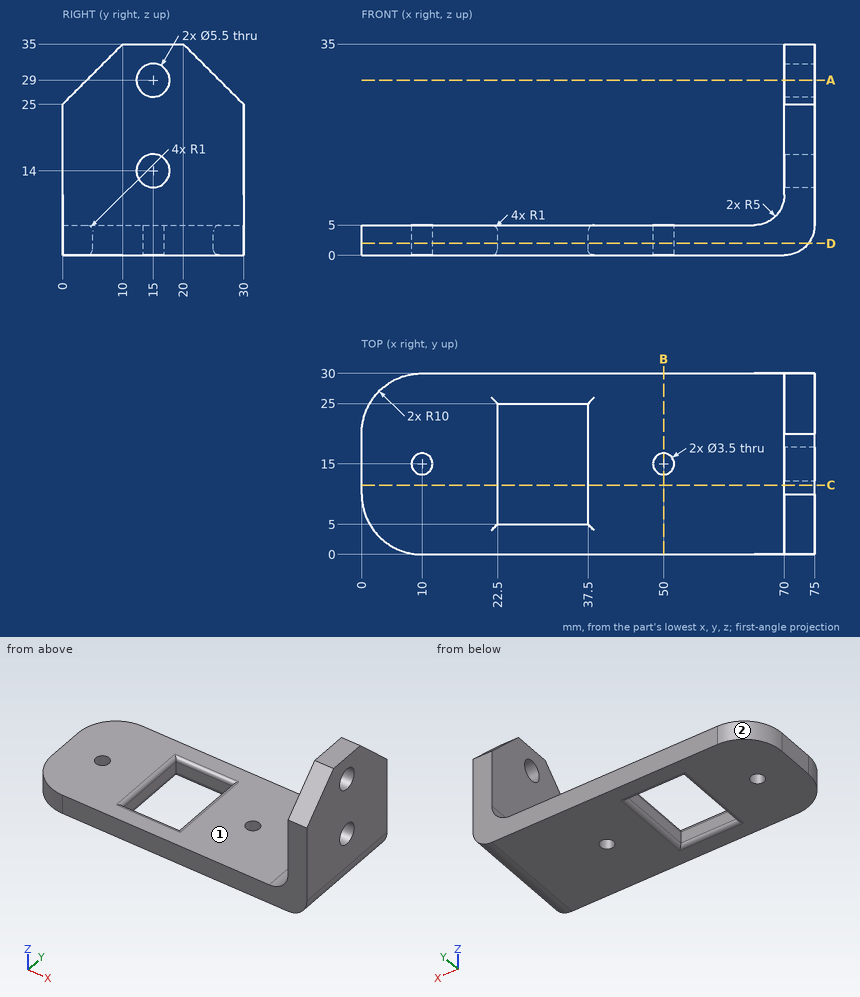
For this review, use the dimensioned drawing (mm, ordinates from the lowest corner) and the shaded views. A direction names the side the tool comes from. Round coordinates to 2 decimals unless told otherwise and drop trailing zeros. Loops run counter-clockwise (first coordinate to the right, second up) from the corner with the lowest first, then second, coordinate; pieces in that order, holes last. Notation, with made-up numbers: (-15, -34.5) -> (-2, -34.5) arc R30 ccw to (-2, -7.5) -> close; hole circle Ø7 at (55.5, 26). An arc over 180 degrees is marked (long way). Write item = value, one per line. Start each with the question number.
Item 1: To check wall thickness, follow L1, parallel to Z at x = 71, y = 15; L2, parallel to Z at x = 48.5, y = 13; L3, parallel to X at y = 27, z = 20. State the ranges of each line that lie inside material, in increasing order.
Item 2: Take a section at C-C on y = 11.5. Give the boundary of the cut face in (x, z), plus the area to 3 significant figures.
Item 3: Take a section at A-A on z = 29. Give the boundary of the cut face in (x, y).
Item 4: Insertion check: pin 1 (8 mm diameter, centred on y = 24, z = 20.5, fed in from -X); pin 2 (4.5 mm diameter, centred on x = 10, y = 15, fed in from +Z); pin 3 (4 mm diameter, centred on x = 38, y = 22, fed in from -Z); pin 4 (2.5 mm diameter, centred on y = 14, z = 2, fed in from +X). Each pin has a flat end and moves straight along its axis. Give the tip position at first contact, or say it passes through.
Item 5: Take a section at D-D on z = 2. Give the boundary of the cut face in (x, y), plus the area to 3 significant figures.
Item 6: For the marked faces 1 and 2, list the 3-axis set-ups (+Z, -Z, +X, -X, +Y, -Y) from which the entire face can be reached by the end or side of a thin tool; tool diameter is ignored.
Item 7: Take a section at B-B on x = 50. Give the boundary of the cut face in (y, z), plus the area to 4 significant figures.
Result:
q1.L1 = 0.1 to 11.25, 16.75 to 26.25, 31.75 to 35
q1.L2 = 0 to 5
q1.L3 = 70 to 75
q2.outline = (0, 0) -> (21.5, 0) arc R1 ccw to (22.5, 1) -> (22.5, 4) arc R1 ccw to (21.5, 5) -> (0, 5) -> close; (37.5, 1) arc R1 ccw to (38.5, 0) -> (70, 0) arc R5 ccw to (75, 5) -> (75, 35) -> (70, 35) -> (70, 10) arc R5 cw to (65, 5) -> (38.5, 5) arc R1 ccw to (37.5, 4) -> close
q2.area = 449 mm²
q3.outline = (70, 4) -> (75, 4) -> (75, 12.25) -> (70, 12.25) -> close; (70, 17.75) -> (75, 17.75) -> (75, 26) -> (70, 26) -> close
q4.pin_1 = 70
q4.pin_2 = 5
q4.pin_3 = 0
q4.pin_4 = 74.68
q5.outline = (0, 10) arc R10 ccw to (10, 0) -> (74, 0) -> (74, 30) -> (10, 30) arc R10 ccw to (0, 20) -> close; hole circle Ø3.5 at (10, 15); hole (22.5, 5) -> (37.5, 5) -> (37.5, 25) -> (22.5, 25) -> close; hole circle Ø3.5 at (50, 15)
q5.area = 1,860 mm²
q6.face_1 = +Z, -X, +Y, -Y
q6.face_2 = +Z, -Z, -X, +Y
q7.outline = (0, 0) -> (13.25, 0) -> (13.25, 5) -> (0, 5) -> close; (16.75, 0) -> (30, 0) -> (30, 5) -> (16.75, 5) -> close
q7.area = 132.5 mm²
